```python
from build123d import *

# Parameters (mm, degrees)
ESBO_O1_R                = 3.5
RESSALTO_EXTRUS_O1_DEPTH = 13
ESBO_O2_R                = 5
RESSALTO_EXTRUS_O2_DEPTH = 57
ESBO_O3_R                = 1.6
CORTE_EXTRUS_O1_DEPTH    = 34


with BuildPart() as part:
    # Esboço1 → Ressalto-extrusão1 (new body)
    with BuildSketch(Plane.XY):
        with BuildLine():
            Line((-10, 0), (-10, 15))
            Line((-10, 15), (10, 15))
            Line((10, 15), (10, 0))
            ThreePointArc((10, 0), (0, -10), (-10, 0))
        make_face()
        with Locations(Location((0, 0, 0), (0, 0, 180))):
            Circle(ESBO_O1_R, mode=Mode.SUBTRACT)
    extrude(amount=RESSALTO_EXTRUS_O1_DEPTH)

    # Esboço2 → Ressalto-extrusão2 (add)
    with BuildSketch(Plane(origin=(0, 15, 0), x_dir=(1, 0, 0), z_dir=(0, 1, 0))):
        with Locations(Location((0, -6.5, 0), (0, 0, 90))):
            Circle(ESBO_O2_R)
    extrude(amount=RESSALTO_EXTRUS_O2_DEPTH)

    # Esboço3 → Corte-extrusão1 (cut)
    with BuildSketch(Plane(origin=(0, 72, 0), x_dir=(1, 0, 0), z_dir=(0, 1, 0))):
        with Locations(Location((0, -6.5, 0), (0, 0, 180))):
            Circle(ESBO_O3_R)
    extrude(amount=-CORTE_EXTRUS_O1_DEPTH, mode=Mode.SUBTRACT)


solid = part.part
```
Geometry check sheet. Reference: the model listing, model coordinates, mm. A direction names the side the tool comes from. Round coordinates to 2 decimals unless told otherwise and drop trailing zeros. Order: outer loops, then holes, each group sorted by start corner. A loop starts at its lowest first (then second) coordinate and runs counter-clockwise, first axis right, second up. Notation, with made-up numbers: (9, 79) - (32, 79) arc R25 cw to (32, 117) - close; hole circle Ø11 at (41.5, -37.75). An arc over 180 degrees is marked (long way). Use a Markdown table: item, result. Add a question column.
(1) Release check for a two-part mould opening along X. For faces 1 (the flat face through (10, 8, 6)), 2 (the flat face through (0, 5, 13)), 3 (the flat face through (0, 38, 7)), 4 (the cylindrical face through (-3.233, 1.341, 6.409)) record: pulls with the +X half, pulls with the -X half, needs draft (parallel to the pull), parting line crosses it, or undercut.
(2) Sectioned sample at C-C, the plane y = 17. Enter the section's corners in (x, z), and give its area (3 significant figures).
(3) Sectioned sample at A-A, the plane x = 0. Enter the section's corners in (y, z), and give its area (3 significant figures).
(4) Material ranges on line 1 along Y through (x, z) = (0, 5.5); line 2 along Y through (x, z) = (0, 10); line 3 along X through (y, z) = (3, 2), recorded low to high. Write a range as [from, to].
(5) Sectioned sample at D-D, the plane z = 6.5. Enter the section's corners in (x, y), and give its area (3 significant figures).
(6) Tool access check on faces 5 (the cylindrical face through (0, -10, 6)), 6 (the cylindrical face through (0.35, 55.24, 4.94)). Record the directions out of +Z, -Z, +X, -X, +Y, -Y that give a thin tool (end or side, any length) a straight path to the whole face; none if there is none.
(7) Sectioned sample at B-B, the plane z = 10.5. Enter the section's corners in (x, y).
(8) Depth check by flat-ended pin: pin 1 (3 mm diameter, centred on x = 0, z = 6.5, fed in from +Y); pin 2 (5 mm diameter, centred on y = 47, z = 4, fed in from +X); pin 3 (2 mm diameter, centred on y = 19, z = 3.5, fed in from -X); pin 4 (12 mm diameter, centred on x = -1.5, y = 11, fed in from -Z). Enter the tip coordinate at first touch or a pass-through.
Answers below:
| question | item | result |
|---|---|---|
| 1 | face 1 | pulls with the +X half |
| 1 | face 2 | needs draft |
| 1 | face 3 | undercut |
| 1 | face 4 | undercut |
| 2 | outline | circle Ø10 at (0, 6.5) |
| 2 | area | 78.5 mm² |
| 3 | outline | (-10, 0) - (-3.5, 0) - (-3.5, 13) - (-10, 13) - close; (3.5, 0) - (15, 0) - (15, 1.5) - (72, 1.5) - (72, 4.9) - (38, 4.9) - (38, 8.1) - (72, 8.1) - (72, 11.5) - (15, 11.5) - (15, 13) - (3.5, 13) - close |
| 3 | area | 695 mm² |
| 4 | line 1 | [-10, -3.5], [3.5, 38] |
| 4 | line 2 | [-10, -3.5], [3.5, 72] |
| 4 | line 3 | [-10, -1.8], [1.8, 10] |
| 5 | outline | (-10, 0) arc R10 ccw to (10, 0) - (10, 15) - (5, 15) - (5, 72) - (1.6, 72) - (1.6, 38) - (-1.6, 38) - (-1.6, 72) - (-5, 72) - (-5, 15) - (-10, 15) - close; hole circle Ø7 at (0, 0) |
| 5 | area | 880 mm² |
| 6 | face 5 | +Z, -Z, -Y |
| 6 | face 6 | +Y |
| 7 | outline | (-10, 0) arc R10 ccw to (10, 0) - (10, 15) - (3, 15) - (3, 72) - (-3, 72) - (-3, 15) - (-10, 15) - close; hole circle Ø7 at (0, 0) |
| 8 | pin 1 | y = 38 |
| 8 | pin 2 | x = 5 |
| 8 | pin 3 | x = -4.58 |
| 8 | pin 4 | z = 0 |
